Could you check a few things on this model? Use its own coordinates, in mm. Round coordinates to 2 decimals unless told otherwise and drop trailing zeros. Write each loop counter-clockwise with the first axis right and the second up, starting at its lowest first coordinate (ties: lowest second). Pieces come first, ordered by that corner, then holes. Notation, with made-up numbers: M 38.25,-18 L 65.25,-18 A11 ccw 65.25,-6 Z; hole C 58,79 d2. An arc over 180 degrees is marked long. One line per item, written item: value. Start each with the question number.
(1) I want a section at B-B on z = 186. Count the separate pieces of the cut face and the enclosed holes in it, and give its area (3 significant figures).
(2) I want a section at A-A on y = 625.5. Please give me the cut outline in (x, z), and give its area (3 significant figures).
(3) If I drill on L1, parallel to Y at x = 1683, z = 625; L2, parallel to Y at x = 1682.5, z = 240; L3, parallel to X at y = 644, z = 460, over which ranges is the centre line in solid material (lowest first)?
(4) I'm going to push flat-ended pins straight in: pin 1 Ø0.5 at (x, z) = (1687.5, 413) entering from +Y; pin 2 Ø4 at (x, z) = (1666, 135) entering from +Y; pin 3 Ø0.8 at (y, z) = (647.5, 344) entering from +X; pin 4 Ø0.5 at (y, z) = (647.5, 514) entering from -X. Where does each tip first touch, or does it pass through?
```python
from build123d import *

# Parameters (mm, degrees)
EXTRUDE_1_DEPTH = 1000


with BuildPart() as part:
    # Model → 凸台-拉伸1 (new body)
    with BuildSketch(Plane.XY):
        with BuildLine():
            Line((1653.86794414, 609.935540563), (1656.86794414, 609.935540563))
            ThreePointArc((1656.86794414, 609.935540563), (1657.026058023, 609.909882212), (1657.16794414, 609.835540563))
            ThreePointArc((1657.16794414, 609.835540563), (1659.86794414, 608.935540563), (1662.56794414, 609.835540563))
            ThreePointArc((1662.56794414, 609.835540563), (1662.709830257, 609.909882212), (1662.86794414, 609.935540563))
            Line((1662.86794414, 609.935540563), (1663.86794414, 609.935540563))
            ThreePointArc((1663.86794414, 609.935540563), (1664.221497531, 609.789093954), (1664.36794414, 609.435540563))
            Line((1664.36794414, 609.435540563), (1664.36794414, 606.435540563))
            ThreePointArc((1664.36794414, 606.435540563), (1664.221497531, 606.081987172), (1663.86794414, 605.935540563))
            Line((1663.86794414, 605.935540563), (1651.36794414, 605.935540563))
            ThreePointArc((1651.36794414, 605.935540563), (1649.953730578, 606.521327001), (1649.36794414, 607.935540563))
            Line((1649.36794414, 607.935540563), (1649.36794414, 645.935540563))
            ThreePointArc((1649.36794414, 645.935540563), (1649.953730578, 647.349754125), (1651.36794414, 647.935540563))
            Line((1651.36794414, 647.935540563), (1663.26794414, 647.935540563))
            Line((1663.26794414, 647.935540563), (1663.26794414, 646.935540563))
            Line((1663.26794414, 646.935540563), (1664.26794414, 646.935540563))
            Line((1664.26794414, 646.935540563), (1664.26794414, 643.935540563))
            Line((1664.26794414, 643.935540563), (1662.26794414, 643.935540563))
            Line((1662.26794414, 643.935540563), (1662.26794414, 644.935540563))
            Line((1662.26794414, 644.935540563), (1660.36794414, 644.935540563))
            ThreePointArc((1660.36794414, 644.935540563), (1659.660837359, 644.642647344), (1659.36794414, 643.935540563))
            Line((1659.36794414, 643.935540563), (1659.36794414, 640.117521078))
            ThreePointArc((1659.36794414, 640.117521078), (1659.444064608, 639.734837646), (1659.660837359, 639.410414297))
            Line((1659.660837359, 639.410414297), (1661.842817874, 637.228433782))
            ThreePointArc((1661.842817874, 637.228433782), (1662.167241223, 637.011661031), (1662.549924656, 636.935540563))
            Line((1662.549924656, 636.935540563), (1676.185963625, 636.935540563))
            ThreePointArc((1676.185963625, 636.935540563), (1676.568647057, 637.011661031), (1676.893070406, 637.228433782))
            Line((1676.893070406, 637.228433782), (1679.075050921, 639.410414297))
            ThreePointArc((1679.075050921, 639.410414297), (1679.291823673, 639.734837646), (1679.36794414, 640.117521078))
            Line((1679.36794414, 640.117521078), (1679.36794414, 643.935540563))
            ThreePointArc((1679.36794414, 643.935540563), (1679.075050921, 644.642647344), (1678.36794414, 644.935540563))
            Line((1678.36794414, 644.935540563), (1676.46794414, 644.935540563))
            Line((1676.46794414, 644.935540563), (1676.46794414, 643.935540563))
            Line((1676.46794414, 643.935540563), (1674.46794414, 643.935540563))
            Line((1674.46794414, 643.935540563), (1674.46794414, 646.935540563))
            Line((1674.46794414, 646.935540563), (1675.46794414, 646.935540563))
            Line((1675.46794414, 646.935540563), (1675.46794414, 647.935540563))
            Line((1675.46794414, 647.935540563), (1687.36794414, 647.935540563))
            ThreePointArc((1687.36794414, 647.935540563), (1688.782157703, 647.349754125), (1689.36794414, 645.935540563))
            Line((1689.36794414, 645.935540563), (1689.36794414, 607.935540563))
            ThreePointArc((1689.36794414, 607.935540563), (1688.782157703, 606.521327001), (1687.36794414, 605.935540563))
            Line((1687.36794414, 605.935540563), (1674.86794414, 605.935540563))
            ThreePointArc((1674.86794414, 605.935540563), (1674.51439075, 606.081987172), (1674.36794414, 606.435540563))
            Line((1674.36794414, 606.435540563), (1674.36794414, 609.435540563))
            ThreePointArc((1674.36794414, 609.435540563), (1674.51439075, 609.789093954), (1674.86794414, 609.935540563))
            Line((1674.86794414, 609.935540563), (1675.86794414, 609.935540563))
            ThreePointArc((1675.86794414, 609.935540563), (1676.026058023, 609.909882212), (1676.16794414, 609.835540563))
            ThreePointArc((1676.16794414, 609.835540563), (1678.86794414, 608.935540563), (1681.56794414, 609.835540563))
            ThreePointArc((1681.56794414, 609.835540563), (1681.709830257, 609.909882212), (1681.86794414, 609.935540563))
            Line((1681.86794414, 609.935540563), (1684.86794414, 609.935540563))
            ThreePointArc((1684.86794414, 609.935540563), (1685.221497531, 610.081987172), (1685.36794414, 610.435540563))
            Line((1685.36794414, 610.435540563), (1685.36794414, 635.218026142))
            ThreePointArc((1685.36794414, 635.218026142), (1684.133311005, 637.065785207), (1681.953730578, 636.632239704))
            Line((1681.953730578, 636.632239704), (1679.721497531, 634.400006657))
            ThreePointArc((1679.721497531, 634.400006657), (1678.099380787, 633.3161429), (1676.185963625, 632.935540563))
            Line((1676.185963625, 632.935540563), (1662.549924656, 632.935540563))
            ThreePointArc((1662.549924656, 632.935540563), (1660.636507494, 633.3161429), (1659.01439075, 634.400006657))
            Line((1659.01439075, 634.400006657), (1656.782157703, 636.632239704))
            ThreePointArc((1656.782157703, 636.632239704), (1654.602577276, 637.065785207), (1653.36794414, 635.218026142))
            Line((1653.36794414, 635.218026142), (1653.36794414, 610.435540563))
            ThreePointArc((1653.36794414, 610.435540563), (1653.51439075, 610.081987172), (1653.86794414, 609.935540563))
        make_face()
        with BuildLine():
            Line((1657.86794414, 639.435540563), (1655.16794414, 639.435540563))
            Line((1655.16794414, 639.435540563), (1655.16794414, 640.435540563))
            Line((1655.16794414, 640.435540563), (1653.56794414, 640.435540563))
            Line((1653.56794414, 640.435540563), (1653.56794414, 639.435540563))
            Line((1653.56794414, 639.435540563), (1650.86794414, 639.435540563))
            Line((1650.86794414, 639.435540563), (1650.86794414, 642.135540563))
            Line((1650.86794414, 642.135540563), (1651.86794414, 642.135540563))
            Line((1651.86794414, 642.135540563), (1651.86794414, 643.735540563))
            Line((1651.86794414, 643.735540563), (1650.86794414, 643.735540563))
            Line((1650.86794414, 643.735540563), (1650.86794414, 645.435540563))
            ThreePointArc((1650.86794414, 645.435540563), (1651.160837359, 646.142647344), (1651.86794414, 646.435540563))
            Line((1651.86794414, 646.435540563), (1653.56794414, 646.435540563))
            Line((1653.56794414, 646.435540563), (1653.56794414, 645.435540563))
            Line((1653.56794414, 645.435540563), (1655.16794414, 645.435540563))
            Line((1655.16794414, 645.435540563), (1655.16794414, 646.435540563))
            Line((1655.16794414, 646.435540563), (1657.86794414, 646.435540563))
            Line((1657.86794414, 646.435540563), (1657.86794414, 643.735540563))
            Line((1657.86794414, 643.735540563), (1656.86794414, 643.735540563))
            Line((1656.86794414, 643.735540563), (1656.86794414, 642.135540563))
            Line((1656.86794414, 642.135540563), (1657.86794414, 642.135540563))
            Line((1657.86794414, 642.135540563), (1657.86794414, 639.435540563))
        make_face(mode=Mode.SUBTRACT)
        with BuildLine():
            Line((1686.86794414, 643.735540563), (1687.86794414, 643.735540563))
            Line((1687.86794414, 643.735540563), (1687.86794414, 645.435540563))
            ThreePointArc((1687.86794414, 645.435540563), (1687.575050921, 646.142647344), (1686.86794414, 646.435540563))
            Line((1686.86794414, 646.435540563), (1685.16794414, 646.435540563))
            Line((1685.16794414, 646.435540563), (1685.16794414, 645.435540563))
            Line((1685.16794414, 645.435540563), (1683.56794414, 645.435540563))
            Line((1683.56794414, 645.435540563), (1683.56794414, 646.435540563))
            Line((1683.56794414, 646.435540563), (1680.86794414, 646.435540563))
            Line((1680.86794414, 646.435540563), (1680.86794414, 643.735540563))
            Line((1680.86794414, 643.735540563), (1681.86794414, 643.735540563))
            Line((1681.86794414, 643.735540563), (1681.86794414, 642.135540563))
            Line((1681.86794414, 642.135540563), (1680.86794414, 642.135540563))
            Line((1680.86794414, 642.135540563), (1680.86794414, 639.435540563))
            Line((1680.86794414, 639.435540563), (1683.56794414, 639.435540563))
            Line((1683.56794414, 639.435540563), (1683.56794414, 640.435540563))
            Line((1683.56794414, 640.435540563), (1685.16794414, 640.435540563))
            Line((1685.16794414, 640.435540563), (1685.16794414, 639.435540563))
            Line((1685.16794414, 639.435540563), (1687.86794414, 639.435540563))
            Line((1687.86794414, 639.435540563), (1687.86794414, 642.135540563))
            Line((1687.86794414, 642.135540563), (1686.86794414, 642.135540563))
            Line((1686.86794414, 642.135540563), (1686.86794414, 643.735540563))
        make_face(mode=Mode.SUBTRACT)
    extrude(amount=EXTRUDE_1_DEPTH)


solid = part.part
```
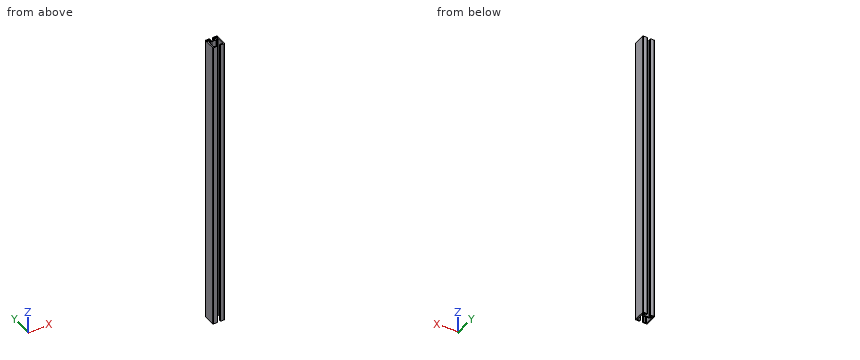
Found:
1. separate pieces: 1
1. enclosed holes: 2
1. area: 586 mm²
2. outline: M 1649.37,0 L 1653.37,0 L 1653.37,1000 L 1649.37,1000 Z; M 1685.37,0 L 1689.37,0 L 1689.37,1000 L 1685.37,1000 Z
2. area: 8,000 mm²
3. L1: y = 605.94 to 609.94, 637.18 to 639.44, 646.44 to 647.94
3. L2: y = 605.94 to 609.94, 637.02 to 639.44, 646.44 to 647.94
3. L3: x = 1649.37 to 1650.87, 1657.87 to 1659.37, 1662.27 to 1664.27, 1674.47 to 1676.47, 1679.37 to 1680.87, 1687.87 to 1689.37
4. pin 1: stops at y = 647.94
4. pin 2: stops at y = 646.94
4. pin 3: stops at x = 1688.99
4. pin 4: stops at x = 1649.86
